```python
from build123d import *

# Parameters (mm, degrees)
BOSS_EXTRUDE1_DEPTH  = 3.175
BOSS_EXTRUDE2_DEPTH  = 3.175
BOSS_EXTRUDE3_START  = -3.175
BOSS_EXTRUDE3_DEPTH  = 6.35
FILLET1_R            = 1.524
FILLET1_OF_MIRROR1_R = 1.524
BOSS_EXTRUDE4_DEPTH  = 0.508


with BuildPart() as part:
    # Sketch1 → Boss-Extrude1 (new body, symmetric)
    with BuildSketch(Plane.XY):
        Polygon((-46.319822715, -26.742762114), (-30.439940905, 0.762), (0, 0.762), (30.439940905, 0.762), (46.319822715, -26.742762114), (15, -26.742762114), (-15, -26.742762114), align=None)
        Polygon((-43.680177285, -25.218762114), (-30, -1.524), (-16.319822715, -25.218762114), align=None, mode=Mode.SUBTRACT)
        Polygon((-28.680177285, -0.762), (-15, -24.456762114), (-1.319822715, -0.762), align=None, mode=Mode.SUBTRACT)
        Polygon((-13.680177285, -25.218762114), (0, -1.524), (13.680177285, -25.218762114), align=None, mode=Mode.SUBTRACT)
        Polygon((1.319822715, -0.762), (15, -24.456762114), (28.680177285, -0.762), align=None, mode=Mode.SUBTRACT)
        Polygon((16.319822715, -25.218762114), (30, -1.524), (43.680177285, -25.218762114), align=None, mode=Mode.SUBTRACT)
    extrude(amount=BOSS_EXTRUDE1_DEPTH, both=True)

    # Sketch2 → Boss-Extrude2 (add, symmetric)
    with BuildSketch(Plane.XY):
        with BuildLine():
            Line((-46.606437051, -27.885762114), (-47.54, -27.885762114))
            Line((-47.54, -27.885762114), (-47.54, -25.218762114))
            Line((-47.54, -25.218762114), (-42.46, -25.218762114))
            Line((-42.46, -25.218762114), (-42.46, -27.885762114))
            Line((-42.46, -27.885762114), (-43.393562949, -27.885762114))
            ThreePointArc((-43.393562949, -27.885762114), (-45, -26.869762114), (-46.606437051, -27.885762114))
        make_face()
        with BuildLine():
            Line((-27.46, 0.762), (-30.439940905, 0.762))
            Line((-30.439940905, 0.762), (-32.54, -2.875409051))
            Line((-32.54, -2.875409051), (-32.54, 0.762))
            Line((-32.54, 0.762), (-32.54, 1.905))
            Line((-32.54, 1.905), (-31.606437051, 1.905))
            ThreePointArc((-31.606437051, 1.905), (-30, 0.889), (-28.393562949, 1.905))
            Line((-28.393562949, 1.905), (-27.46, 1.905))
            Line((-27.46, 1.905), (-27.46, 0.762))
        make_face()
        with BuildLine():
            Line((-16.606437051, -27.885762114), (-17.54, -27.885762114))
            Line((-17.54, -27.885762114), (-17.54, -26.742762114))
            Line((-17.54, -26.742762114), (-12.46, -26.742762114))
            Line((-12.46, -26.742762114), (-12.46, -27.885762114))
            Line((-12.46, -27.885762114), (-13.393562949, -27.885762114))
            ThreePointArc((-13.393562949, -27.885762114), (-15, -26.869762114), (-16.606437051, -27.885762114))
        make_face()
    boss_extrude2 = extrude(amount=BOSS_EXTRUDE2_DEPTH, both=True)

    # Sketch3 → Boss-Extrude3 (add)
    with BuildSketch(Plane.XY.offset(BOSS_EXTRUDE3_START)):
        with BuildLine():
            Line((1.606437051, 1.905), (2.54, 1.905))
            Line((2.54, 1.905), (2.54, 0.762))
            Line((2.54, 0.762), (-2.54, 0.762))
            Line((-2.54, 0.762), (-2.54, 1.905))
            Line((-2.54, 1.905), (-1.606437051, 1.905))
            ThreePointArc((-1.606437051, 1.905), (0, 0.889), (1.606437051, 1.905))
        make_face()
    extrude(amount=BOSS_EXTRUDE3_DEPTH)

    # Fillet1
    fillet1_edges = [part.edges().sort_by_distance(p)[0] for p in [
        (-47.54, -25.218762114, 0),
    ]]
    fillet(fillet1_edges, radius=FILLET1_R)

    # Mirror1: Boss-Extrude2 across plane
    add(boss_extrude2.mirror(Plane(origin=(0, 0, 0), x_dir=(0, 0, 1), z_dir=(1, 0, 0))))

    # Fillet1 of Mirror1
    fillet1_of_mirror1_edges = [part.edges().sort_by_distance(p)[0] for p in [
        (47.54, -25.218762114, 0),
    ]]
    fillet(fillet1_of_mirror1_edges, radius=FILLET1_OF_MIRROR1_R)

    # Sketch4 → Boss-Extrude4 (add)
    with BuildSketch(Plane(origin=(30.341470111, 0.762, -10.998323426), x_dir=(-1, 0, 0), z_dir=(0, 1, 0))):
        Polygon((55.766638301, 8.903049935), (54.0821519, 8.903049935), (54.924395101, 13.184452869), (56.608881501, 13.184452869), align=None)
        with BuildLine():
            Line((49.373679321, 8.903049935), (51.695796166, 13.184452869))
            Line((51.695796166, 13.184452869), (53.731217234, 13.184452869))
            Line((53.731217234, 13.184452869), (53.455071922, 11.780714202))
            Line((53.455071922, 11.780714202), (52.044845481, 11.780714202))
            ThreePointArc((52.044845481, 11.780714202), (51.895660414, 11.763021636), (51.754751921, 11.710925494))
            ThreePointArc((51.754751921, 11.710925494), (50.74099205, 10.52746368), (50.853552966, 8.973236868))
            Line((50.853552966, 8.973236868), (50.888554794, 8.903049935))
            Line((50.888554794, 8.903049935), (49.373679321, 8.903049935))
        make_face()
        with BuildLine():
            Line((47.344206299, 13.184452869), (47.92473551, 8.903049935))
            Line((47.92473551, 8.903049935), (45.657455804, 8.903049935))
            Line((45.657455804, 8.903049935), (45.800093765, 8.973236868))
            ThreePointArc((45.800093765, 8.973236868), (46.559919921, 9.999679495), (46.16385217, 11.213784347))
            ThreePointArc((46.16385217, 11.213784347), (46.087708374, 11.278047887), (46.002485287, 11.329668676))
            ThreePointArc((46.002485287, 11.329668676), (45.241879319, 11.641820064), (44.44239948, 11.833632247))
            ThreePointArc((44.44239948, 11.833632247), (44.321830206, 11.897125178), (44.264573877, 12.020777977))
            ThreePointArc((44.264573877, 12.020777977), (44.273299822, 12.151811254), (44.326168164, 12.272022736))
            ThreePointArc((44.326168164, 12.272022736), (44.436687002, 12.409847066), (44.584321098, 12.50687352))
            ThreePointArc((44.584321098, 12.50687352), (45.07356558, 12.617554773), (45.566896159, 12.526805434))
            ThreePointArc((45.566896159, 12.526805434), (45.796502387, 12.340831934), (45.882880346, 12.05826511))
            Line((45.882880346, 12.05826511), (45.882880346, 11.780714202))
            Line((45.882880346, 11.780714202), (46.993271632, 11.780714202))
            ThreePointArc((46.993271632, 11.780714202), (47.00184458, 12.512372899), (46.712523898, 13.184452869))
            Line((46.712523898, 13.184452869), (47.344206299, 13.184452869))
        make_face()
        with BuildLine():
            Line((52.362572033, 10.727910202), (53.247962938, 10.727910202))
            Line((53.247962938, 10.727910202), (53.040853955, 9.675106202))
            Line((53.040853955, 9.675106202), (52.224130208, 9.675106202))
            ThreePointArc((52.224130208, 9.675106202), (51.949800938, 9.788737106), (51.836170033, 10.063066377))
            Line((51.836170033, 10.063066377), (51.836170033, 10.201508202))
            ThreePointArc((51.836170033, 10.201508202), (51.990349609, 10.573730626), (52.362572033, 10.727910202))
        make_face()
        Polygon((48.958505766, 10.596309702), (48.845492907, 11.429779536), (49.410557201, 11.429779536), align=None)
        Polygon((48.607571099, 13.184452869), (50.362244433, 13.184452869), (50.019637029, 12.552770469), (48.69322295, 12.552770469), align=None)
        with BuildLine():
            Line((43.093358174, 9.007864255), (43.203837606, 8.897384823))
            Line((43.203837606, 8.897384823), (41.238603472, 8.897384823))
            ThreePointArc((41.238603472, 8.897384823), (42.59037643, 10.850382179), (42.150373231, 13.184452869))
            Line((42.150373231, 13.184452869), (43.624298831, 13.184452869))
            ThreePointArc((43.624298831, 13.184452869), (42.976922737, 12.00046329), (43.609533036, 10.808518937))
            ThreePointArc((43.609533036, 10.808518937), (43.801404112, 10.703005905), (44.00849344, 10.63186155))
            Line((44.00849344, 10.63186155), (45.137184548, 10.349688773))
            ThreePointArc((45.137184548, 10.349688773), (45.325274084, 10.217067986), (45.375126192, 9.992388851))
            ThreePointArc((45.375126192, 9.992388851), (45.276758726, 9.771226443), (45.079326395, 9.631192719))
            ThreePointArc((45.079326395, 9.631192719), (44.392498989, 9.682709209), (43.976922089, 10.231964773))
            Line((43.976922089, 10.231964773), (42.853931155, 10.231964773))
            ThreePointArc((42.853931155, 10.231964773), (42.786913393, 9.583390951), (43.093358174, 9.007864255))
        make_face()
        with BuildLine():
            Line((38.57083963, 8.903049935), (36.605605496, 8.903049935))
            ThreePointArc((36.605605496, 8.903049935), (38.014670833, 10.833118693), (37.588222563, 13.184452869))
            Line((37.588222563, 13.184452869), (39.342895896, 13.184452869))
            ThreePointArc((39.342895896, 13.184452869), (38.831372076, 12.513225905), (38.57083963, 11.710527269))
            Line((38.57083963, 11.710527269), (39.693830563, 11.710527269))
            ThreePointArc((39.693830563, 11.710527269), (39.959617235, 12.233880985), (40.415270694, 12.603910164))
            ThreePointArc((40.415270694, 12.603910164), (41.166876497, 12.593701608), (41.591788981, 11.973649288))
            ThreePointArc((41.591788981, 11.973649288), (41.543037796, 10.949193829), (41.155213354, 9.999731945))
            ThreePointArc((41.155213354, 9.999731945), (40.782487914, 9.571566118), (40.251107207, 9.371854393))
            ThreePointArc((40.251107207, 9.371854393), (39.531077174, 9.674914925), (39.41308283, 10.447162469))
            Line((39.41308283, 10.447162469), (38.149718029, 10.447162469))
            ThreePointArc((38.149718029, 10.447162469), (38.201808334, 9.631886976), (38.57083963, 8.903049935))
        make_face()
        with BuildLine():
            Line((35.48104333, 9.602571887), (35.356873428, 9.602571887))
            ThreePointArc((35.356873428, 9.602571887), (34.923728887, 9.759646665), (34.691948891, 10.157848515))
            ThreePointArc((34.691948891, 10.157848515), (34.675735454, 10.986379145), (34.920455715, 11.778110082))
            ThreePointArc((34.920455715, 11.778110082), (35.261440878, 12.213116508), (35.747757566, 12.475790357))
            ThreePointArc((35.747757566, 12.475790357), (35.911443016, 12.505405638), (36.077655631, 12.511990293))
            ThreePointArc((36.077655631, 12.511990293), (36.647671195, 12.253324316), (36.864077445, 11.665962276))
            ThreePointArc((36.864077445, 11.665962276), (36.699639375, 10.801331502), (36.294750409, 10.019864179))
            ThreePointArc((36.294750409, 10.019864179), (35.938277424, 9.712977507), (35.48104333, 9.602571887))
        make_face()
    extrude(amount=BOSS_EXTRUDE4_DEPTH)


solid = part.part
```
Could you check a few things on this model? Use its own coordinates, in mm. A direction names the side the tool comes from. Round coordinates to 2 decimals unless told otherwise and drop trailing zeros. Write each loop counter-clockwise with the first axis right and the second up, starting at its lowest first coordinate (ties: lowest second). Pieces come first, ordered by that corner, then holes. Notation, with made-up numbers: M 60,21.25 L 111,21.25 A15 ccw 111,41.25 Z; hole C 21,72 d7. An arc over 180 degrees is marked long. Write each question's results on one line, items separated by ' | '. Start each with the question number.
1. Thinking about a two-plate mould opening in X: for faces 1 (the face through (32.54, -1, 0)), 2 (the face through (-20.18, 1.01, 0.02)), 3 (the face through (-47.11, -25.68, -0.04)), 4 (the face through (30.03, 0.89, -0.04)), which applies, +X half, -X half, draft (parallel to the pull), parting line (faces both ways), or undercut?
2. Imagine slicing it at C-C on x = 26.5. List the corners of the cut face in (y, z) for me (3 decimals), and give its area (3 significant figures).
3. I'm going to push flat-ended pins straight in: pin 1 Ø3 at (x, z) = (-20.5, -1.5) entering from -Y; pin 2 Ø12 at (x, y) = (-13, -7) entering from +Z; pin 3 Ø2.5 at (y, z) = (-0.5, 1.5) entering from -X; pin 4 Ø2 at (x, z) = (-22, 0.5) entering from +Y. Where does each tip first touch, or does it pass through?
4. I need wall thicknesses on L1, parallel to X at y = -13.75, z = 1.5; L2, parallel to Y at x = -4, z = 0.25; L3, parallel to Y at x = -20, z = -2. Which ranges of each line are inside material? Lowest first, please. Write a range as from..to.
5. On a 3-axis mill with a long thin cutter (end or side, diameter ignored), from which of +Z, -Z, +X, -X, +Y, -Y can I reach the whole of each face in a straight line? I mean faces 5 (the face through (-30, -25.219, 0)), 6 (the face through (44.97, -26.87, -0.04)), 7 (the face through (-32.54, -1, 0)). Say none if no direction works.
6. Imagine slicing it at B-B on x = -38.5. List the corners of the cut face in (y, z) for me (3 decimals), and give its area (3 significant figures).
7. Imagine slicing it at A-A on y = -8. List the corners of the cut face in (x, z) for me (3 decimals).
Result sheet:
1) face 1: +X half | face 2: undercut | face 3: -X half | face 4: undercut
2) outline: M -26.743,-3.175 L -25.219,-3.175 L -25.219,3.175 L -26.743,3.175 Z; M -7.586,-3.175 L -4.538,-3.175 L -4.538,3.175 L -7.586,3.175 Z; M -0.762,-3.175 L 0.762,-3.175 L 0.762,3.175 L -0.762,3.175 Z | area: 38.7 mm^2
3) pin 1: stops at y = -26.74 | pin 2: passes through | pin 3: stops at x = -32.54 | pin 4: stops at y = 1.27
4) L1: x = -38.82..-37.06, -22.94..-21.18, -8.82..-7.06, 7.06..8.82, 21.18..22.94, 37.06..38.82 | L2: y = -26.74..-25.22, -8.45..-5.4, -0.76..0.76 | L3: y = -26.74..-25.22, -18.84..-15.8, -0.76..1.27
5) face 5: +Z, -Z | face 6: +Z, -Z, -Y | face 7: +Z, -Z, -X, +Y
6) outline: M -26.743,-3.175 L -25.219,-3.175 L -25.219,3.175 L -26.743,3.175 Z; M -16.246,-3.175 L -13.198,-3.175 L -13.198,3.175 L -16.246,3.175 Z | area: 29.0 mm^2
7) outline: M -35.499,-3.175 L -33.739,-3.175 L -33.739,3.175 L -35.499,3.175 Z; M -26.261,-3.175 L -24.501,-3.175 L -24.501,3.175 L -26.261,3.175 Z; M -5.499,-3.175 L -3.739,-3.175 L -3.739,3.175 L -5.499,3.175 Z; M 3.739,-3.175 L 5.499,-3.175 L 5.499,3.175 L 3.739,3.175 Z; M 24.501,-3.175 L 26.261,-3.175 L 26.261,3.175 L 24.501,3.175 Z; M 33.739,-3.175 L 35.499,-3.175 L 35.499,3.175 L 33.739,3.175 Z
